Solid Edge part; units mm, degrees
sketch "Sketch1" plane through (0, 0, 0) normal (0, 0, 1) x (1, 0, 0)
  line L0 (-3, 3) -> (-3, 0)
  line L1 (-3, 0) -> (-9, 0)
  line L2 (-9, 0) -> (-9, 10)
  line L3 (-9, 10) -> (9, 10)
  line L4 (9, 10) -> (9, 0)
  line L5 (9, 0) -> (3, 0)
  line L6 (3, 3) -> (3, 0)
  arc A0 (3, 3) -> (-3, 3) centre (0, 3) ccw
  dimension "D1" = 9
  dimension "D2" = 3
  dimension "D3" = 9
extrude "Protrusion1" add sketch "Sketch1" along normal mid plane 18
sketch "Sketch2" plane through (0, 10, 0) normal (0, 1, 0) x (1, 0, 0)
  circle A0 centre (-5, 5) radius 1.7
  dimension "D1" = 5
extrude "Cutout1" cut sketch "Sketch2" against normal through all
mirror "Mirror1" about plane through (0, 0, 0) normal (1, 0, 0) of "Cutout1"
mirror "Mirror2" about plane through (0, 0, 0) normal (0, 0, 1) of "Cutout1", "Mirror1"
properties material "ABS Plastic, high impact"
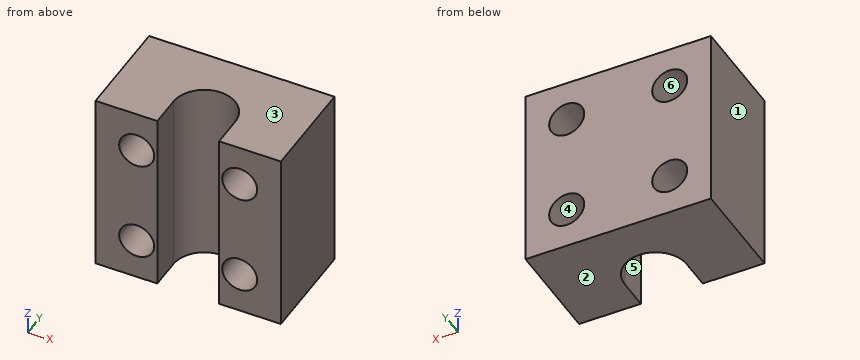
Work out the finished part from the listing and answer in its coordinate system (mm). Face numbers are marked on the shaded views. A direction names the side the tool comes from. Coordinates: 2 decimals unless noted, no trailing zeros. Order: outer loops, then holes, each group sorted by start corner. A loop starts at its lowest first (then second) coordinate and runs counter-clockwise, first axis right, second up. Notation, with made-up numbers: M -12,5 L 11,5 A25 cw 11,38 Z; hole C 38.5,15.25 d8. An arc over 180 degrees is marked long. Use CSV: the item, a comma, the result in double quotes.
1) Section D-D on y = 8 is taken. Write down the section's boundary in (x, z), plus the area to 3 significant figures.
Worked out:
outline,"M -9,-9 L 9,-9 L 9,9 L -9,9 Z; hole C -5,-5 d3.4; hole C -5,5 d3.4; hole C 5,-5 d3.4; hole C 5,5 d3.4"
area,"288 mm^2"
2) A flat-ended cylindrical pin translates along its axis: pin 1 Ø2 at (x, z) = (-5, 5) entering from -Y. Find the tip coordinate at first contact, or state that the pin passes through.
Worked out:
pin 1,"passes through"
3) Determine the mould class of the marked faces 1, 2, 3 and 4 for opening direction Z: released by +Z, released by -Z, zero draft, split by the parting line, or undercut.
Worked out:
face 1,"zero draft"
face 2,"released by -Z"
face 3,"released by +Z"
face 4,"undercut"
4) For the marked faces 5 and 6, determine the directions among +Z, -Z, +X, -X, +Y, -Y from which every point of the face is accessible in a straight line to the end or side of a thin tool.
Worked out:
face 5,"+Z, -Z, -Y"
face 6,"+Y, -Y"
5) Section B-B on z = 5 is taken. Write down the section's boundary in (x, y), plus the area to 3 significant figures.
Worked out:
outline,"M -9,0 L -6.7,0 L -6.7,10 L -9,10 Z; M -3.3,0 L -3,0 L -3,3 A3 cw 3,3 L 3,0 L 3.3,0 L 3.3,10 L -3.3,10 Z; M 6.7,0 L 9,0 L 9,10 L 6.7,10 Z"
area,"79.9 mm^2"
6) Section A-A on y = 1.5 is taken. Write down the section's boundary in (x, z).
Worked out:
outline,"M -9,-9 L -3,-9 L -3,9 L -9,9 Z; M 3,-9 L 9,-9 L 9,9 L 3,9 Z; hole C -5,-5 d3.4; hole C -5,5 d3.4; hole C 5,-5 d3.4; hole C 5,5 d3.4"
7) Consider line 1 (Z direction, x = 5, y = 3.75); line 2 (X direction, y = 2, z = -5); line 3 (X direction, y = 0.75, z = 2). Determine where each line is inside the solid, lowest interval first. Write a range as [from, to].
Worked out:
line 1,"z = [-9, -6.7], [-3.3, 3.3], [6.7, 9]"
line 2,"x = [-9, -6.7], [-3.3, -3], [3, 3.3], [6.7, 9]"
line 3,"x = [-9, -3], [3, 9]"
8) Section C-C on x = -5 is taken. Write down the section's boundary in (y, z), plus the area to 3 significant figures.
Worked out:
outline,"M 0,-9 L 10,-9 L 10,-6.7 L 0,-6.7 Z; M 0,-3.3 L 10,-3.3 L 10,3.3 L 0,3.3 Z; M 0,6.7 L 10,6.7 L 10,9 L 0,9 Z"
area,"112 mm^2"
